Autodesk Inventor part; units mm, degrees
ref_plane "YZ Plane" through (0, 0, 0) normal (1, 0, 0) x (0, 1, 0)
ref_plane "XZ Plane" through (0, 0, 0) normal (0, 1, 0) x (-1, 0, 0)
ref_plane "XY Plane" through (0, 0, 0) normal (0, 0, 1) x (1, 0, 0)
sketch "Sketch1" plane through (0, 0, 0) normal (1, 0, 0) x (0, 1, 0)
  line L0 (0, 0) -> (203.2, 0)
  line L1 (203.2, 0) -> (203.2, -203.2)
  line L2 (203.2, -203.2) -> (0, -203.2)
  line L3 (0, -203.2) -> (0, 0)
  dimension "d0" = 203.2
  dimension "d1" = 203.2
extrude "Extrusion1" add sketch "Sketch1" along normal blind 457.2
shell "Shell1" thickness 8.636 removed faces 0
properties part number "CinderBlock" material "Concrete"
Check sheet for the modelled part. Datum: model origin and axes. Units: mm. A direction names the side the tool comes from. Coordinates: 2 decimals unless noted, no trailing zeros. Loops run counter-clockwise (first coordinate to the right, second up) from the corner with the lowest first, then second, coordinate; pieces in that order, holes last. Notation, with made-up numbers: M 49.25,73 L 107.25,73 A11 ccw 107.25,89 Z; hole C 51,85 d3. An arc over 180 degrees is marked long. Answer as a JSON object with one key per item and string values.
1. Sectioned sample at B-B on x = 58. Record the cut outline in (y, z), and give its area (3 significant figures).
Outcome:
{"outline": "M 0,-203.2 L 203.2,-203.2 L 203.2,0 L 0,0 Z; hole M 8.64,-194.56 L 194.56,-194.56 L 194.56,-8.64 L 8.64,-8.64 Z", "area": "6,720 mm²"}
2. Scan lines: L1, parallel to Z at x = 380, y = 91; L2, parallel to Y at x = 226, z = -133; L3, parallel to X at y = 19, z = -68.5. Record each from-to range of solid material in increasing order. Write a range as from..to.
Outcome:
{"L1": "-203.2..-194.56, -8.64..0", "L2": "0..8.64, 194.56..203.2", "L3": "0..8.64, 448.56..457.2"}
3. Release check for a two-part mould opening along Z. For faces 3 (the flat face through (226, 8.636, -103)), 4 (the flat face through (448.564, 100, -100)), 5 (the flat face through (225, 103, -203.2)), 6 (the flat face through (225, 203.2, -100)) record: pulls with the +Z half, pulls with the -Z half, needs draft (parallel to the pull), parting line crosses it, or undercut.
Outcome:
{"face 3": "undercut", "face 4": "undercut", "face 5": "pulls with the -Z half", "face 6": "needs draft"}
4. Sectioned sample at A-A on z = -66. Record the cut outline in (x, y).
Outcome:
{"outline": "M 0,0 L 457.2,0 L 457.2,203.2 L 0,203.2 Z; hole M 8.64,8.64 L 448.56,8.64 L 448.56,194.56 L 8.64,194.56 Z"}
5. Access from +Z, -Z, +X, -X, +Y, -Y to the whole of each face (thin tool, end or side, straight path). Record for faces 1 (the flat face through (457.2, 100, -100)), 2 (the flat face through (8.636, 100, -100)).
Outcome:
{"face 1": "+Z, -Z, +X, +Y, -Y", "face 2": "none"}
